from build123d import *

# Parameters (mm, degrees)
F1_DEPTH = 17
F2_R     = 1.8
F3_DEPTH = 7
F4_R     = 1.8
F5_DEPTH = 7
F6_R     = 1.8
F7_DEPTH = 12


with BuildPart() as f1:
    # F0 (on Right) → F1 (new body, symmetric)
    with BuildSketch(Plane.YZ):
        with BuildLine():
            Line((-140, 0), (0, 0))
            Line((0, 0), (0, 7))
            Line((0, 7), (-125.860693, 7))
            ThreePointArc((-125.860693, 7), (-133.749292, 5.15419), (-140, 0))
        make_face()
    extrude(amount=F1_DEPTH, both=True)

    # F2 (on face) → F3 (cut)
    with BuildSketch(Plane.YZ.offset(17)):
        with Locations((-20, 3.5)):
            Circle(F2_R)
        with Locations((-120, 3.5)):
            Circle(F2_R)
    extrude(amount=-F3_DEPTH, mode=Mode.SUBTRACT)

    # F4 (on face) → F5 (cut)
    with BuildSketch(Plane(origin=(-17, 0, 0), x_dir=(0, -1, 0), z_dir=(-1, 0, 0))):
        with Locations((20, 3.5)):
            Circle(F4_R)
        with Locations((120, 3.5)):
            Circle(F4_R)
    extrude(amount=-F5_DEPTH, mode=Mode.SUBTRACT)

    # F6 (on face) → F7 (cut)
    with BuildSketch(Plane(origin=(0, 0, 0), x_dir=(-1, 0, 0), z_dir=(0, 1, 0))):
        with Locations((0, 3.5)):
            Circle(F6_R)
    extrude(amount=-F7_DEPTH, mode=Mode.SUBTRACT)


solid = f1.part
Source: CAD feature listing. Evaluate the final solid. Frame: model axes, mm. A direction names the side the tool comes from. Give positions to 0.01 mm unless a question says otherwise; leave off trailing zeros. Write each loop counter-clockwise with the first axis right and the second up, starting at its lowest first coordinate (ties: lowest second). Pieces come first, ordered by that corner, then holes. Notation, with made-up numbers: M 8.5,62 L 59.5,62 A36 cw 59.5,100 Z; hole C 64.5,6.5 d5. An arc over 180 degrees is marked long. Answer as a JSON object with one key per item and string values.
Q1. Access query for faces 4 (the face through (-13.549, -19.766, 5.285)), 5 (the face through (0, -12, 4)), 6 (the face through (0.238, -133.647, 5.205)), 7 (the face through (13.549, -20.234, 5.285)). Directions: +Z, -Z, +X, -X, +Y, -Y. A direction counts if a zero-diameter tool reaches every point of the face in a straight line with its end or side. Return the directions, or none.
Geometry check:
{"face 4": "-X", "face 5": "+Y", "face 6": "+Z, +X, -X, -Y", "face 7": "+X"}
Q2. Cut plane A-A, the plane x = 14.5. Return the cut outline in (y, z).
Geometry check:
{"outline": "M -140,0 L 0,0 L 0,7 L -125.86,7 A17.78 ccw Z; hole C -120,3.5 d3.6; hole C -20,3.5 d3.6"}
Q3. Cut plane D-D, the plane z = 3.5. Return the cut outline in (x, y).
Geometry check:
{"outline": "M -17,-136.45 L 17,-136.45 L 17,-121.8 L 10,-121.8 L 10,-118.2 L 17,-118.2 L 17,-21.8 L 10,-21.8 L 10,-18.2 L 17,-18.2 L 17,0 L 1.8,0 L 1.8,-12 L -1.8,-12 L -1.8,0 L -17,0 L -17,-18.2 L -10,-18.2 L -10,-21.8 L -17,-21.8 L -17,-118.2 L -10,-118.2 L -10,-121.8 L -17,-121.8 Z"}
Q4. Ray query, line 1 along Z through (x, y) = (13.25, -120); line 2 along Y through (x, z) = (-15, 3.25); line 3 along Y through (x, z) = (-12, 2). Return the intervals inside material, ascending.
Geometry check:
{"line 1": "z = 0 to 1.7, 5.3 to 7", "line 2": "y = -136.78 to -121.78, -118.22 to -21.78, -18.22 to 0", "line 3": "y = -138.22 to -120.99, -119.01 to -20.99, -19.01 to 0"}
Q5. Cut plane B-B, the plane y = -120. Return the cut outline in (x, z), then the cut area to 3 significant figures.
Geometry check:
{"outline": "M -17,0 L 17,0 L 17,1.7 L 10,1.7 L 10,5.3 L 17,5.3 L 17,7 L -17,7 L -17,5.3 L -10,5.3 L -10,1.7 L -17,1.7 Z", "area": "188 mm^2"}
Q6. Contact query for flat-ended pins moving along their axis: P1, Ø3, axis at y = -120, z = 3.5, coming from the +X side; P2, Ø3, axis at x = 0, z = 3.5, coming from the +Y side; P3, Ø2, axis at x = 2.5, z = 4.5, coming from the -Y side. Output: stop coordinate, or through.
Geometry check:
{"P1": "stops at x = 10", "P2": "stops at y = -12", "P3": "stops at y = -136.45"}
Q7. Cut plane C-C, the plane x = 0. Return the cut outline in (y, z), then the cut area to 3 significant figures.
Geometry check:
{"outline": "M -140,0 L 0,0 L 0,1.7 L -12,1.7 L -12,5.3 L 0,5.3 L 0,7 L -125.86,7 A17.78 ccw Z", "area": "907 mm^2"}
Q8. Mould query, pull axis Z, two halves, no side actions, for faces 1 (the face through (0, -62, 7)), 2 (the face through (17, -71, 4)), 3 (the face through (13.55, -121.8, 3.58)). Classes: +Z half, -Z half, draft (parallel to the pull), parting line (faces both ways), or undercut.
Geometry check:
{"face 1": "+Z half", "face 2": "draft", "face 3": "undercut"}
